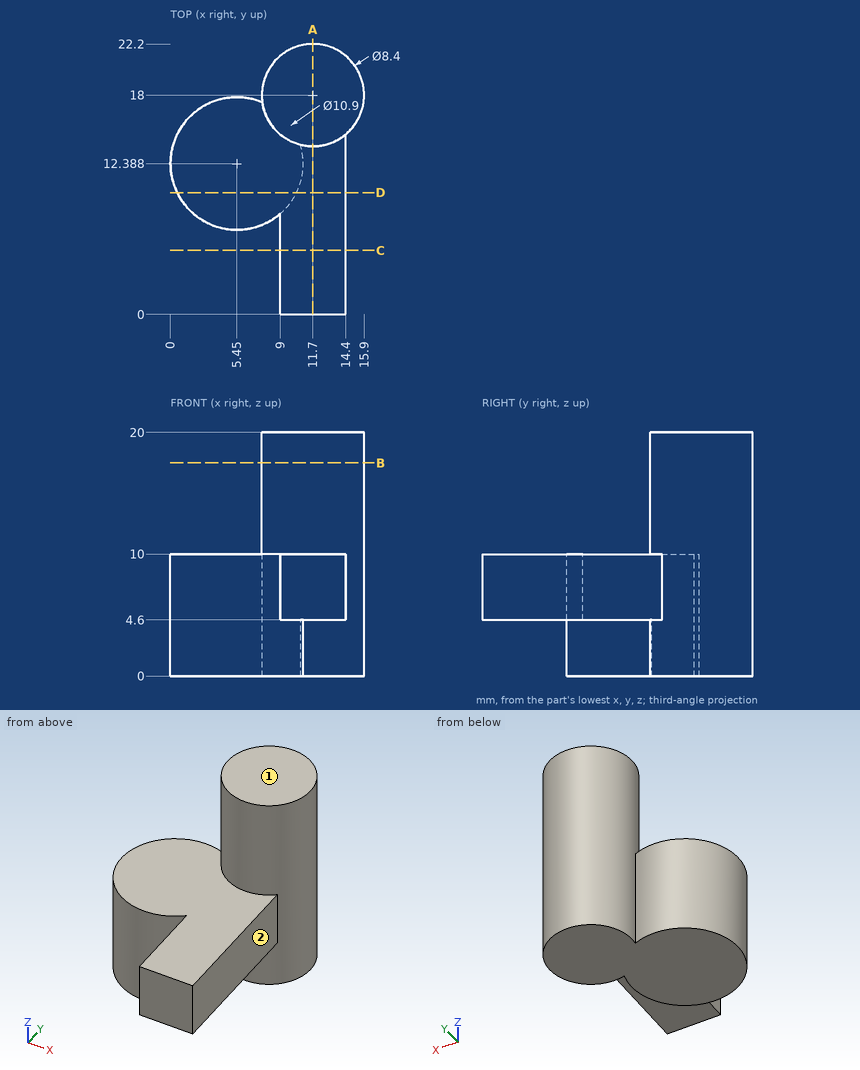
Could you check a few things on this drawing? It's one solid part, dimensions in mm from its lowest x, y, z. A direction names the side the tool comes from. Round coordinates to 2 decimals unless told otherwise and drop trailing zeros. Write each loop counter-clockwise with the first axis right and the second up, starting at its lowest first coordinate (ties: lowest second). Pieces come first, ordered by that corner, then holes.
Q1. Please list where these lines run through material, in increasing order: probe 1 along Z at (x, y) = (11.5, 5.5); probe 2 along X at (y, z) = (6.75, 7); probe 3 along Z at (x, y) = (8.5, 12).
Q2. If we section it at C-C on y = 5.25: Write out the boundary of the cut face in (x, z).
Q3. If we section it at A-A on x = 11.7: Write out the boundary of the cut face in (y, z).
Q4. Will these pins go through, and if not, where does the flat tip stop? P1, Ø6, axis at y = 3, z = 7.5, coming from the -X side; P2, Ø10, axis at y = 6, z = 12.5, coming from the +X side; P3, Ø2.5, axis at x = 12.5, y = 8.5, coming from the -Z side.
Q5. If we section it at D-D on y = 10: Write out the boundary of the cut face in (x, z).
Q6. Which directions (+Z, -Z, +X, -X, +Y, -Y) give clear straight access to the entire face, cutting with the end or side of a thin tool? Please do the marked faces 1 and 2.
Q7. If we section it at B-B on z = 17.5: Write out the boundary of the cut face in (x, y).
Answer below:
1. probe 1: z = 4.6 to 10
1. probe 2: x = 9 to 14.4
1. probe 3: z = 0 to 10
2. outline: (9, 4.6) - (14.4, 4.6) - (14.4, 10) - (9, 10) - close
3. outline: (0, 4.6) - (13.8, 4.6) - (13.8, 0) - (22.2, 0) - (22.2, 20) - (13.8, 20) - (13.8, 10) - (0, 10) - close
4. P1: stops at x = 9
4. P2: stops at x = 14.4
4. P3: stops at z = 4.6
5. outline: (0.55, 0) - (10.35, 0) - (10.35, 4.6) - (14.4, 4.6) - (14.4, 10) - (0.55, 10) - close
6. face 1: +Z, +X, -X, +Y, -Y
6. face 2: +Z, -Z, +X, -Y
7. outline: circle Ø8.4 at (11.7, 18)
